Read the model definition and answer for the solid it produces. Units are mm, in the model's axes. Face numbers are marked on the shaded views. Coordinates: 2 decimals unless noted, no trailing zeros. Write each loop counter-clockwise with the first axis right and the second up, starting at its lowest first coordinate (ties: lowest second). Pieces come first, ordered by that corner, then holes.
1) Determine the mould class of the marked faces 1, 2 and 3 for opening direction X: +X half, -X half, draft (parallel to the pull), parting line (faces both ways), or undercut.
2) The part is cut by section B-B (y = -19.75). Determine the outline of the cut face in (x, z), then the cut area to 3 significant figures.
3) Find the intervals of material crossed by line 1 (Z direction, x = -49.5, y = -24); line 2 (X direction, y = -6.75, z = -21); line 3 (Z direction, x = -1, y = -13.75), in increasing order.
4) Each of these flat-tipped pins is pushed along its axis until it touches: pin 1 Ø10 at (x, y) = (14, -13) entering from +Z; pin 2 Ø12 at (x, y) = (-51, -7) entering from +Z; pin 3 Ø1.1 at (y, z) = (-12, 2) entering from -X. Where does it stop, or does it pass through?
5) The part is cut by section A-A (x = 40). Determine the outline of the cut face in (y, z), then the cut area to 3 significant figures.
6) The part is cut by section C-C (z = -20). Determine the outline of the cut face in (x, y), then the cut area to 3 significant figures.
7) The part is cut by section D-D (x = -53.5). Determine the outline of the cut face in (y, z).
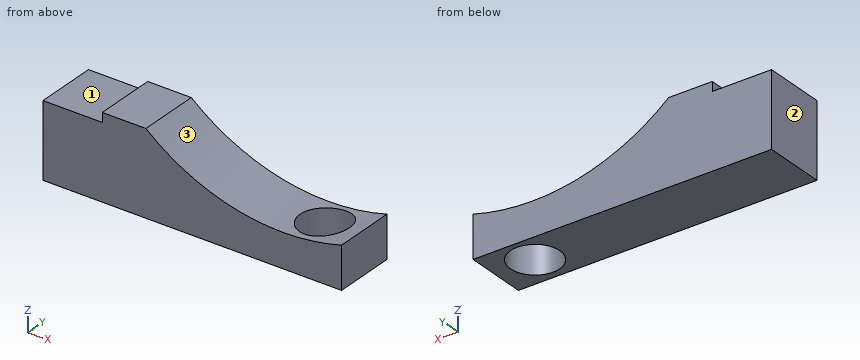
from build123d import *

# Parameters (mm, degrees)
F1_DEPTH = 25.4
F3_D     = 20.32


with BuildPart() as f1:
    # F0 (on Front) → F1 (new body)
    with BuildSketch(Plane.XZ):
        with BuildLine():
            Line((-68.265416, 0), (-68.265416, -30.535927))
            Line((-68.265416, -30.535927), (54.465521, -30.535927))
            Line((54.465521, -30.535927), (54.465521, -13.212661))
            ThreePointArc((54.465521, -13.212661), (12.125602, -14.688008), (-25.9849, 3.816991))
            Line((-25.9849, 3.816991), (-43.895394, 3.816991))
            Line((-43.895394, 3.816991), (-43.895394, 0))
            Line((-43.895394, 0), (-68.265416, 0))
        make_face()
    extrude(amount=F1_DEPTH)

    # F3 (through all)
    with Locations(Plane.XY):
        with Locations((38.023103, -12.331817)):
            Hole(F3_D / 2)


solid = f1.part
Reported:
1. face 1: draft
1. face 2: -X half
1. face 3: undercut
2. outline: (-68.27, -30.54) - (31.08, -30.54) - (31.08, -16.59) arc R87.88 cw to (-25.98, 3.82) - (-43.9, 3.82) - (-43.9, 0) - (-68.27, 0) - close; (44.97, -30.54) - (54.47, -30.54) - (54.47, -13.21) arc R87.88 cw to (44.97, -15.37) - close
2. area: 2,670 mm2
3. line 1: z = -30.54 to 0
3. line 2: x = -68.27 to 29.53, 46.51 to 54.47
3. line 3: z = -30.54 to -10.82
4. pin 1: stops at z = -13.97
4. pin 2: stops at z = 0
4. pin 3: stops at x = -43.9
5. outline: (-25.4, -30.54) - (-22.3, -30.54) - (-22.3, -16.06) - (-25.4, -16.06) - close; (-2.37, -30.54) - (0, -30.54) - (0, -16.06) - (-2.37, -16.06) - close
5. area: 79.2 mm2
6. outline: (-68.27, -25.4) - (54.47, -25.4) - (54.47, 0) - (-68.27, 0) - close; hole circle Ø20.32 at (38.02, -12.33)
6. area: 2,790 mm2
7. outline: (-25.4, -30.54) - (0, -30.54) - (0, 0) - (-25.4, 0) - close
